Can you work these out from the model? Positions are in its coordinate system, mm. Face numbers are marked on the shaded views. A direction names the side the tool comes from. Round coordinates to 2 decimals unless told otherwise and drop trailing zeros. Loops run counter-clockwise (first coordinate to the right, second up) from the corner with the lowest first, then second, coordinate; pieces in that order, holes last. Notation, with made-up numbers: M 38.5,59 L 58.5,59 A32 ccw 58.5,92 Z; hole C 4,-8.75 d11. An arc over 180 degrees is marked long. Return JSON: item names as keys, results as strings.
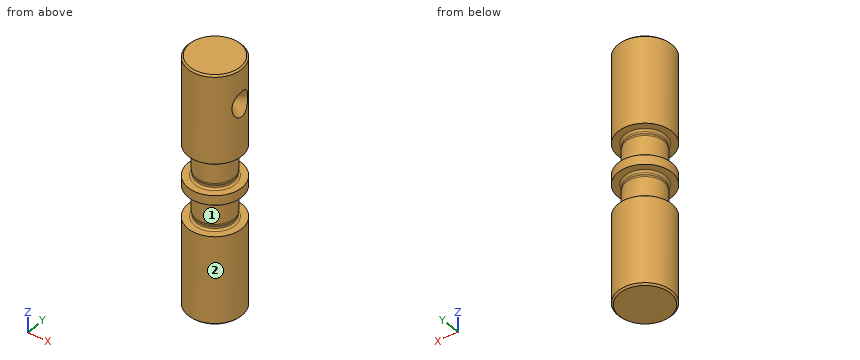
```python
from build123d import *

# Parameters (mm, degrees)
F4_SIZE = 0.5


with BuildPart() as f1:
    # F0 (on Front) → F1 (revolve)
    with BuildSketch(Plane.XZ):
        with BuildLine():
            Line((-8.5, 0), (0, 0))
            Line((0, 0), (0, 79))
            Line((0, 79), (-8.5, 79))
            Line((-8.5, 79), (-8.5, 51))
            Line((-8.5, 51), (-6.4, 51))
            ThreePointArc((-6.4, 51), (-5.975736, 50.824264), (-5.8, 50.4))
            Line((-5.8, 50.4), (-5.8, 49.825402))
            ThreePointArc((-5.8, 49.825402), (-5.805133, 49.747086), (-5.820445, 49.67011))
            Line((-5.820445, 49.67011), (-6, 49))
            Line((-6, 49), (-6, 43))
            Line((-6, 43), (-5.820445, 42.32989))
            ThreePointArc((-5.820445, 42.32989), (-5.805133, 42.252914), (-5.8, 42.174598))
            Line((-5.8, 42.174598), (-5.8, 41.6))
            ThreePointArc((-5.8, 41.6), (-5.975736, 41.175736), (-6.4, 41))
            Line((-6.4, 41), (-8.5, 41))
            Line((-8.5, 41), (-8.5, 38))
            Line((-8.5, 38), (-6.4, 38))
            ThreePointArc((-6.4, 38), (-5.975736, 37.824264), (-5.8, 37.4))
            Line((-5.8, 37.4), (-5.8, 36.825402))
            ThreePointArc((-5.8, 36.825402), (-5.805133, 36.747086), (-5.820445, 36.67011))
            Line((-5.820445, 36.67011), (-6, 36))
            Line((-6, 36), (-6, 30))
            Line((-6, 30), (-5.820445, 29.32989))
            ThreePointArc((-5.820445, 29.32989), (-5.805133, 29.252914), (-5.8, 29.174598))
            Line((-5.8, 29.174598), (-5.8, 28.6))
            ThreePointArc((-5.8, 28.6), (-5.975736, 28.175736), (-6.4, 28))
            Line((-6.4, 28), (-8.5, 28))
            Line((-8.5, 28), (-8.5, 0))
        make_face()
    revolve(axis=Axis((0, 0, 39.5), (0, 0, -1)))

    # F2 (on Front) → F3 (revolve, cut)
    with BuildSketch(Plane.XZ):
        Polygon((8.5, 67.5), (8.5, 71.5), (4.5, 67.5), align=None)
    revolve(axis=Axis((1.375147, 0, 67.5), (1, 0, 0)), mode=Mode.SUBTRACT)

    # F4
    f4_edges = [f1.edges().sort_by_distance(p)[0] for p in [
        (8.5, 0, 79),
        (8.5, 0, 0),
    ]]
    chamfer(f4_edges, length=F4_SIZE)


solid = f1.part
```
Q1. On a 3-axis mill with a long thin cutter (end or side, diameter ignored), from which of +Z, -Z, +X, -X, +Y, -Y can I reach the whole of each face in a straight line? I mean the marked faces 1 and 2. Say none if no direction works.
Results:
{"face 1": "none", "face 2": "+Z, -Z"}
Q2. I'm going to push flat-ended pins straight in: pin 1 Ø5 at (y, z) = (3, 10.5) entering from -X; pin 2 Ø6 at (x, z) = (-4, 57) entering from -Y; pin 3 Ø2 at (x, z) = (-6.5, 8) entering from +Y. Where does each tip first touch, or does it pass through?
Results:
{"pin 1": "stops at x = -8.49", "pin 2": "stops at y = -8.44", "pin 3": "stops at y = 6.48"}
Q3. If I drill on line 1 along Z through (x, y) = (-0.5, 7.5); line 2 along Y through (x, z) = (0.5, 22); line 3 along Z through (x, y) = (-6, 1), over which ranges is the centre line in solid material (lowest first)?
Results:
{"line 1": "z = 0 to 28, 38 to 41, 51 to 79", "line 2": "y = -8.49 to 8.49", "line 3": "z = 0 to 28.09, 37.91 to 41.09, 50.91 to 79"}
Q4. Suppose I cut it at A-A, the plane z = 73.5. Please give me the cut outline in (x, y).
Results:
{"outline": "C 0,0 d17"}
